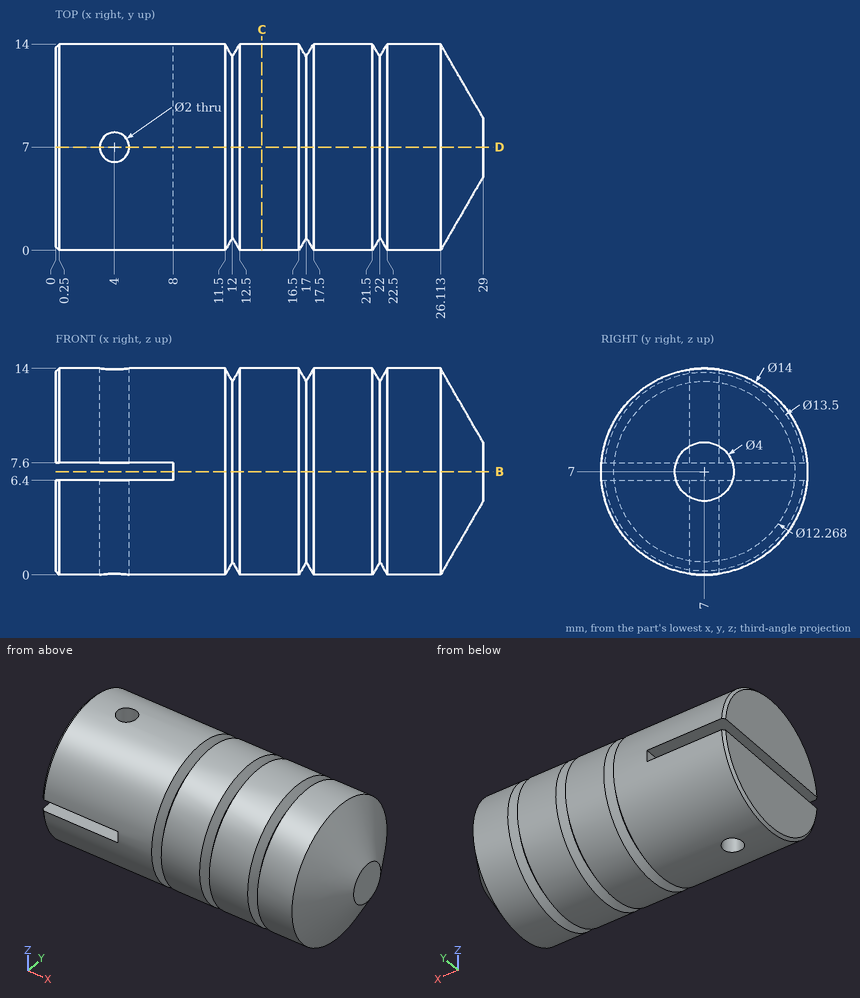
The figure shows three views and two pictorial views of one solid part (mm, origin at its lowest corner). Answer the questions. Give positions to 0.01 mm unless a question says otherwise; leave off trailing zeros. Order: outer loops, then holes, each group sorted by start corner. A loop starts at its lowest first (then second) coordinate and runs counter-clockwise, first axis right, second up. Notation, with made-up numbers: (63.25, -20.75) -> (118.25, -20.75) arc R24 cw to (118.25, -4.75) -> close; hole circle Ø9 at (-32.75, 69.25). An arc over 180 degrees is marked (long way). Answer as a JSON object with one key per item and string values. Group by question number.
Item 1: The part is cut by section D-D on y = 7. Give the number of separate pieces and of enclosed holes in the cut face, and give its area (3 significant figures).
Item 2: The part is cut by section B-B on z = 7. Write down the section's boundary in (x, y).
Item 3: Flat-ended cylindrical pins translate along their axes: pin 1 (2 mm diameter, centred on x = 15.5, z = 2.5, fed in from +Y); pin 2 (3 mm diameter, centred on x = 4, y = 7, fed in from -Z); pin 3 (1 mm diameter, centred on y = 11, z = 6, fed in from +X); pin 4 (6 mm diameter, centred on x = 25, z = 2.5, fed in from -Y). Find the tip coordinate at first contact, or state that the pin passes through.
Item 4: The part is cut by section C-C on x = 14. Write down the section's boundary in (y, z).
Item 5: Consider L1, parallel to Y at x = 4.75, z = 2.5; L2, parallel to Y at x = 4, z = 9.25; L3, parallel to X at y = 7.25, z = 8. Determine where each line is inside the solid, lowest interval first. Write a range as from..to.
Result set:
{
 "1": {"separate pieces": "3", "enclosed holes": "0", "area": "354 mm²"},
 "2": {"outline": "(8, 0) -> (11.5, 0) -> (12, 0.87) -> (12.5, 0) -> (16.5, 0) -> (17, 0.87) -> (17.5, 0) -> (21.5, 0) -> (22, 0.87) -> (22.5, 0) -> (26.11, 0) -> (29, 5) -> (29, 9) -> (26.11, 14) -> (22.5, 14) -> (22, 13.13) -> (21.5, 14) -> (17.5, 14) -> (17, 13.13) -> (16.5, 14) -> (12.5, 14) -> (12, 13.13) -> (11.5, 14) -> (8, 14) -> close"},
 "3": {"pin 1": "y = 13.06", "pin 2": "z = 0", "pin 3": "x = 28.06", "pin 4": "y = 0.16"},
 "4": {"outline": "circle Ø14 at (7, 7)"},
 "5": {"L1": "1.64..6.34, 7.66..12.36", "L2": "0.37..6, 8..13.63", "L3": "0..3.03, 4.97..29"}
}
